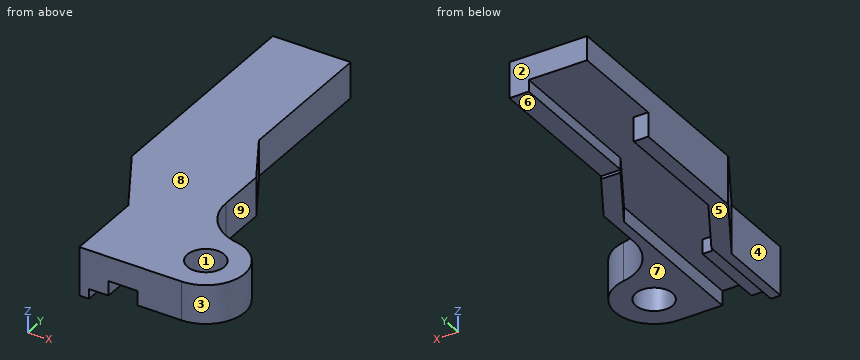
from build123d import *

# Parameters (mm, degrees)
SKETCH_1_R          = 1.9
EXTRUDE_1_DEPTH     = 4
SKETCH_2_W          = 3
SKETCH_2_H          = 1.5
CUT_EXTRUDE_1_DEPTH = 14.793114224
SKETCH_3_W          = 1
SKETCH_3_H          = 8
EXTRUDE_2_DEPTH     = 1
SKETCH_4_W          = 5.5
SKETCH_4_H          = 30
EXTRUDE_3_DEPTH     = 2.5
EXTRUDE_4_DEPTH     = 15
SKETCH_6_W          = 2
SKETCH_6_H          = 1.2
EXTRUDE_5_DEPTH     = 15
EXTRUDE_6_REACH     = 37.672
CUT_EXTRUDE_2_REACH = 37.809
EXTRUDE_7_DEPTH     = 2.5
EXTRUDE_8_REACH     = 39.047
SKETCH_11_W         = 1.5
SKETCH_11_H         = 10
CUT_EXTRUDE_3_DEPTH = 2.5
CUT_EXTRUDE_4_REACH = 35.56
SKETCH_12_W         = 1
SKETCH_12_H         = 1
FILLET_1_R          = 5


with BuildPart() as part:
    # 草图1 → 凸台-拉伸1 (new body)
    with BuildSketch(Plane.XY):
        with BuildLine():
            Line((0, 4), (-10.5, 4))
            Line((-10.5, 4), (-10.5, -4))
            Line((-10.5, -4), (0, -4))
            ThreePointArc((0, -4), (4, 0), (0, 4))
        make_face()
        Circle(SKETCH_1_R, mode=Mode.SUBTRACT)
    extrude(amount=EXTRUDE_1_DEPTH)

    # 草图2 → 切除-拉伸1 (cut, through all)
    with BuildSketch(Plane(origin=(0, 4, 0), x_dir=(1, 0, 0), z_dir=(0, 1, 0))):
        with Locations((-6, -0.75)):
            Rectangle(SKETCH_2_W, SKETCH_2_H)
    extrude(amount=-CUT_EXTRUDE_1_DEPTH, mode=Mode.SUBTRACT)

    # 草图3 → 凸台-拉伸2 (add)
    with BuildSketch(Plane(origin=(0, 0, 0), x_dir=(-1, 0, 0), z_dir=(0, 0, -1))):
        with Locations((10, 0)):
            Rectangle(SKETCH_3_W, SKETCH_3_H)
    extrude(amount=EXTRUDE_2_DEPTH)

    # 草图4 → 凸台-拉伸3 (add)
    with BuildSketch(Plane.XY.offset(4)):
        with Locations((-7.75, 19)):
            Rectangle(SKETCH_4_W, SKETCH_4_H)
    extrude(amount=-EXTRUDE_3_DEPTH)

    # 草图5 → 凸台-拉伸4 (add)
    with BuildSketch(Plane(origin=(0, 4, 0), x_dir=(1, 0, 0), z_dir=(0, 1, 0))):
        Polygon((-5, -4), (-3.5, -4), (-3.5, 0), (-4.5, 0), (-4.5, -1.5), (-5, -1.5), align=None)
    extrude(amount=EXTRUDE_4_DEPTH)

    # 草图6 → 凸台-拉伸5 (add)
    with BuildSketch(Plane(origin=(0, 19, 0), x_dir=(1, 0, 0), z_dir=(0, 1, 0))):
        with Locations((-7.5, -0.9)):
            Rectangle(SKETCH_6_W, SKETCH_6_H)
    extrude(amount=EXTRUDE_5_DEPTH)

    # 凸台-拉伸6: up to this face of the body (flat: up to its plane)
    extrude_6_end = Plane(part.part.faces().sort_by_distance((-8.5, 0, 0))[0])
    # 草图7 → 凸台-拉伸6 (add, up to the picked face)
    with BuildSketch(Plane(origin=(0, 0, 1.5), x_dir=(-1, 0, 0), z_dir=(0, 0, -1)), mode=Mode.PRIVATE) as extrude_6_sk1:
        Polygon((8.5, 19), (4.5, 12.07179677), (4.5, 19), align=None)
    extrude_6_tool1 = split(extrude(extrude_6_sk1.sketch, amount=EXTRUDE_6_REACH, mode=Mode.PRIVATE), bisect_by=extrude_6_end, keep=Keep.BOTH, mode=Mode.PRIVATE)
    add(extrude_6_tool1.solids().sort_by(Axis((-5.833333, 16.690599, 1.5), (0, 0, -1)))[0])

    # 草图8 → 切除-拉伸2 (cut, up to next)
    with BuildSketch(Plane(origin=(0, 0, 0), x_dir=(-1, 0, 0), z_dir=(0, 0, -1)), mode=Mode.PRIVATE) as cut_extrude_2_sk1:
        Polygon((6.5, 34), (6.5, 19), (3.5, 13.803847577), (3.5, 19), (5, 19), (5, 34), align=None)
    cut_extrude_2_tool1 = extrude(cut_extrude_2_sk1.sketch, amount=-CUT_EXTRUDE_2_REACH, mode=Mode.PRIVATE) & part.part
    add(cut_extrude_2_tool1.solids().sort_by_distance((-5.428395, 24.124739, 0))[0], mode=Mode.SUBTRACT)

    # 草图9 → 凸台-拉伸7 (add)
    with BuildSketch(Plane.XY.offset(4)):
        Polygon((-10.5, 34), (-14.5, 34), (-14.5, 10.92820323), (-10.5, 4), align=None)
    extrude(amount=-EXTRUDE_7_DEPTH)

    # 凸台-拉伸8: up to this face of the body (flat: up to its plane)
    extrude_8_end = Plane(part.part.faces().sort_by_distance((-10, 0, -1))[0])
    # 草图10 → 凸台-拉伸8 (add, up to the picked face)
    with BuildSketch(Plane(origin=(0, 0, 1.5), x_dir=(-1, 0, 0), z_dir=(0, 0, -1)), mode=Mode.PRIVATE) as extrude_8_sk1:
        Polygon((8.5, 4), (13, 11.794228634), (13, 34), (14.5, 34), (14.5, 10.92820323), (10.5, 4), align=None)
    extrude_8_tool1 = split(extrude(extrude_8_sk1.sketch, amount=EXTRUDE_8_REACH, mode=Mode.PRIVATE), bisect_by=extrude_8_end, keep=Keep.BOTH, mode=Mode.PRIVATE)
    add(extrude_8_tool1.solids().sort_by(Axis((-13.105485, 18.144493, 1.5), (0, 0, -1)))[0])

    # 草图11 → 切除-拉伸3 (cut)
    with BuildSketch(Plane(origin=(0, 0, -1), x_dir=(-1, 0, 0), z_dir=(0, 0, -1))):
        with Locations((13.75, 29)):
            Rectangle(SKETCH_11_W, SKETCH_11_H)
    extrude(amount=-CUT_EXTRUDE_3_DEPTH, mode=Mode.SUBTRACT)

    # 切除-拉伸4: up to this face of the body (flat: up to its plane)
    cut_extrude_4_end = Plane(part.part.faces().sort_by_distance((-10.75, 7.897114317, 0.25))[0])
    # 草图12 → 切除-拉伸4 (cut, up to the picked face)
    with BuildSketch(Plane.XZ.offset(-4), mode=Mode.PRIVATE) as cut_extrude_4_sk1:
        with Locations((-9, -0.5)):
            Rectangle(SKETCH_12_W, SKETCH_12_H)
    cut_extrude_4_tool1 = split(extrude(cut_extrude_4_sk1.sketch, amount=-CUT_EXTRUDE_4_REACH, mode=Mode.PRIVATE), bisect_by=cut_extrude_4_end, keep=Keep.BOTH, mode=Mode.PRIVATE)
    add(cut_extrude_4_tool1.solids().sort_by(Axis((-9, 4, -0.5), (0, 1, 0)))[0], mode=Mode.SUBTRACT)

    # 圆角1
    fillet_1_edges = [part.edges().sort_by_distance(p)[0] for p in [
        (-3.5, 4, 2),
    ]]
    fillet(fillet_1_edges, radius=FILLET_1_R)


solid = part.part
The model under review builds one solid part; all positions refer to its coordinate system, in mm. Face numbers are marked on the shaded views. A direction names the side the tool comes from. Coordinates: 2 decimals unless noted, no trailing zeros. Loops run counter-clockwise (first coordinate to the right, second up) from the corner with the lowest first, then second, coordinate; pieces in that order, holes last.
(1) Draft analysis for pull direction X (two halves, no side actions). For the marked faces 1, 2, 3 and 4, state which applies: +X half, -X half, draft (parallel to the pull), parting line (faces both ways), or undercut.
Determined:
face 1: undercut
face 2: draft
face 3: +X half
face 4: -X half
(2) Wall thickness on L1, parallel to X at y = -1, z = 0.6; L2, parallel to Z at x = -3.25, y = 3.5; L3, parallel to Y at x = 0, z = 1.95: over which ranges is each line inside the solid? List them lowest first.
Determined:
L1: x = -10.5 to -7.5, -4.5 to -1.62, 1.62 to 3.87
L2: z = 0 to 4
L3: y = -4 to -1.9, 1.9 to 4.1
(3) Consider section A-A, the plane y = 0. Give the boundary of the cut face in (x, z), plus the area to 3 significant figures.
Determined:
outline: (-10.5, -1) - (-9.5, -1) - (-9.5, 0) - (-7.5, 0) - (-7.5, 1.5) - (-4.5, 1.5) - (-4.5, 0) - (-1.9, 0) - (-1.9, 4) - (-10.5, 4) - close; (1.9, 0) - (4, 0) - (4, 4) - (1.9, 4) - close
area: 39.3 mm2
(4) Insertion check: P1, Ø2, axis at x = -8, y = 2.5, coming from the -Z side; P2, Ø0.8, axis at y = 20, z = -0.5, coming from the +X side; P3, Ø0.8, axis at x = -14, z = 0.5, coming from the +Y side. Each pin has a flat end and moves straight along its axis. Give the tip position at first contact, or say it passes through.
Determined:
P1: stops at z = 0
P2: stops at x = -13
P3: stops at y = 24
(5) Consider section B-B, the plane z = -0.5. Give the boundary of the cut face in (x, y), plus the area to 3 significant figures.
Determined:
outline: (-14.5, 10.93) - (-10.5, 4) - (-10.5, -4) - (-9.5, -4) - (-9.5, 5.73) - (-13, 11.79) - (-13, 24) - (-14.5, 24) - close
area: 40.8 mm2
(6) Consider section C-C, the plane y = 20. Give the boundary of the cut face in (x, z), plus the area to 4 significant figures.
Determined:
outline: (-14.5, -1) - (-13, -1) - (-13, 1.5) - (-8.5, 1.5) - (-8.5, 0.3) - (-6.5, 0.3) - (-6.5, 4) - (-14.5, 4) - close
area: 26.15 mm2
(7) Tool access review of the marked faces 5, 6, 7, 8 and 9: name each direction out of +Z, -Z, +X, -X, +Y, -Y from which nothing blocks a thin tool from reaching the whole face with its end or side.
Determined:
face 5: -Z, +X, -X, +Y, -Y
face 6: -Z, +X, +Y
face 7: -Z, +X, +Y, -Y
face 8: +Z, +X, -X, +Y, -Y
face 9: +Z, -Z, +X, +Y
(8) Consider section D-D, the plane x = -8. Give the boundary of the cut face in (y, z), plus the area to 3 significant figures.
Determined:
outline: (-4, 0) - (4, 0) - (4, 1.5) - (18.13, 1.5) - (18.13, 0) - (19, 0) - (19, 0.3) - (34, 0.3) - (34, 4) - (-4, 4) - close
area: 126 mm2
